Input: part model. Units: mm. Frame: model coordinates. Face numbers are marked on the shaded views. Give positions to 0.01 mm unless a question says otherwise; leave off trailing zeros. Write each loop counter-clockwise with the first axis right and the second up, starting at its lowest first coordinate (ties: lowest second). Pieces come first, ordered by that corner, then holes. Notation, with made-up numbers: (66, -24) -> (77, -24) arc R15 ccw to (77, -12) -> close; hole circle Ø9 at (38, 18.5). An arc over 180 degrees is marked (long way). Return JSON: item names as keys, results as strings. Group by question number.
Item 1: Mould query, pull axis Y, two halves, no side actions, for the marked faces 1 and 2. Classes: released by +Y, released by -Y, zero draft, split by the parting line, or undercut.
Item 2: Section A-A, the plane z = 7.5. Return loops of the section in (x, y).
Item 3: Pin query (flat end, axial travel): P1, Ø5, axis at x = 10, z = 7.5, coming from the +Y side; P2, Ø9.5, axis at x = 10, z = 7.5, coming from the +Y side; P3, Ø2, axis at x = 75, y = -33.5, coming from the -Z side. Return the tip coordinate at first contact, or that it passes through.
Item 4: Section C-C, the plane y = -52. Return loops of the section in (x, z), then the cut area to 3 significant figures.
Item 5: Section B-B, the plane x = 257. Return loops of the section in (y, z).
Item 6: Line query: line 1 (X direction, y = -0.5, z = 7.5); line 2 (Y direction, x = 302, z = 1); line 3 (Z direction, x = 300.5, y = -59). Output: solid intervals per line, ascending. Write a range as [from, to].
from build123d import *

# Parameters (mm, degrees)
SM_BASE_FLANGE_2_DEPTH = 400
SKETCH_15_R            = 3
CUT_EXTRUDE_2_DEPTH    = 411.075127263


# Sheet-metal steps are written as plain solids
with BuildPart() as part:
    # Эскиз9 → Базовая кромка2 (new body)
    with BuildSketch(Plane(origin=(0, 0, 0), x_dir=(0, 0, -1), z_dir=(1, 0, 0))):
        with BuildLine():
            Line((0, 0), (-16, 0))
            ThreePointArc((-16, 0), (-18.828427125, -1.171572875), (-20, -4))
            Line((-20, -4), (-20, -84.1))
            ThreePointArc((-20, -84.1), (-18.828427125, -86.928427125), (-16, -88.1))
            Line((-16, -88.1), (0, -88.1))
            Line((0, -88.1), (0, -86.1))
            Line((0, -86.1), (-16, -86.1))
            ThreePointArc((-16, -86.1), (-17.414213562, -85.514213562), (-18, -84.1))
            Line((-18, -84.1), (-18, -4))
            ThreePointArc((-18, -4), (-17.414213562, -2.585786438), (-16, -2))
            Line((-16, -2), (0, -2))
            Line((0, -2), (0, 0))
        make_face()
    extrude(amount=SM_BASE_FLANGE_2_DEPTH)

    # Эскиз15 → Вырез-Вытянуть2 (cut, through all)
    with BuildSketch(Plane(origin=(0, 0, 0), x_dir=(1, 0, 0), z_dir=(0, 1, 0))):
        with Locations(Location((390, -7.5, 0), (0, 0, 270))):
            Circle(SKETCH_15_R)
        with Locations(Location((10, -7.5, 0), (0, 0, 270))):
            Circle(SKETCH_15_R)
    extrude(amount=-CUT_EXTRUDE_2_DEPTH, mode=Mode.SUBTRACT)


solid = part.part
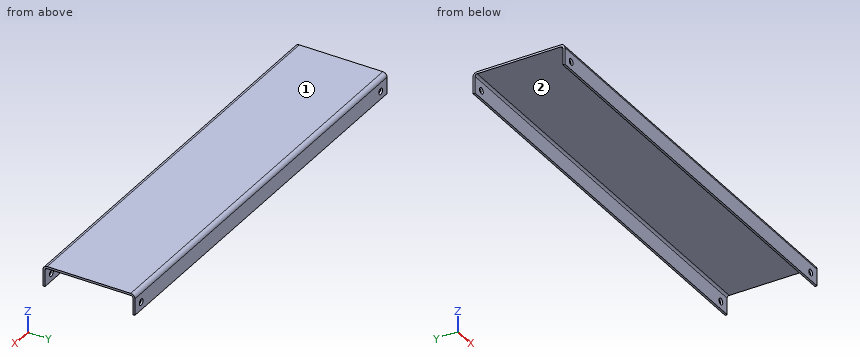
Answer below:
{
 "1": {"face 1": "zero draft", "face 2": "undercut"},
 "2": {"outline": "(0, -88.1) -> (7, -88.1) -> (7, -86.1) -> (0, -86.1) -> close; (0, -2) -> (7, -2) -> (7, 0) -> (0, 0) -> close; (13, -88.1) -> (387, -88.1) -> (387, -86.1) -> (13, -86.1) -> close; (13, -2) -> (387, -2) -> (387, 0) -> (13, 0) -> close; (393, -88.1) -> (400, -88.1) -> (400, -86.1) -> (393, -86.1) -> close; (393, -2) -> (400, -2) -> (400, 0) -> (393, 0) -> close"},
 "3": {"P1": "passes through", "P2": "stops at y = 0", "P3": "stops at z = 18"},
 "4": {"outline": "(0, 18) -> (400, 18) -> (400, 20) -> (0, 20) -> close", "area": "800 mm2"},
 "5": {"outline": "(-88.1, 0) -> (-86.1, 0) -> (-86.1, 16) arc R2 cw to (-84.1, 18) -> (-4, 18) arc R2 cw to (-2, 16) -> (-2, 0) -> (0, 0) -> (0, 16) arc R4 ccw to (-4, 20) -> (-84.1, 20) arc R4 ccw to (-88.1, 16) -> close"},
 "6": {"line 1": "x = [0, 7], [13, 387], [393, 400]", "line 2": "y = [-88.1, -86.1], [-2, 0]", "line 3": "z = [18, 20]"}
}
